CAD build for the part. Positions are in the model's coordinates, mm. Face numbers are marked on the shaded views. A direction names the side the tool comes from. Coordinates: 2 decimals unless noted, no trailing zeros. Loops run counter-clockwise (first coordinate to the right, second up) from the corner with the lowest first, then second, coordinate; pieces in that order, holes last. Notation, with made-up numbers: (54, 41.5) -> (76, 41.5) arc R23 cw to (76, 54.5) -> close; hole circle Ø10 at (64.5, 50.5). An arc over 180 degrees is marked (long way). Write each question's results on one line, items separated by ' | '.
from build123d import *

# Parameters (mm, degrees)
SKETCH_1_W          = 60
SKETCH_1_H          = 44
EXTRUDE_1_DEPTH     = 10
SKETCH_2_W          = 30
SKETCH_2_H          = 36
EXTRUDE_2_DEPTH     = 18
SKETCH_3_R          = 10
CUT_EXTRUDE_1_DEPTH = 47.561786907
RIB_1_REACH         = 48.562
SKETCH_5_WALL_W     = 123.548914622
SKETCH_5_WALL_H     = 6


with BuildPart() as part:
    # 草图1 → 凸台-拉伸1 (new body)
    with BuildSketch(Plane(origin=(0, 0, 0), x_dir=(1, 0, 0), z_dir=(0, 1, 0))):
        Rectangle(SKETCH_1_W, SKETCH_1_H)
    extrude(amount=EXTRUDE_1_DEPTH)

    # 草图2 → 凸台-拉伸2 (add)
    with BuildSketch(Plane(origin=(0, 10, 0), x_dir=(1, 0, 0), z_dir=(0, 1, 0))):
        with Locations((-7, 0)):
            Rectangle(SKETCH_2_W, SKETCH_2_H)
    extrude(amount=EXTRUDE_2_DEPTH)

    # 草图3 → 切除-拉伸1 (cut, through all)
    with BuildSketch(Plane(origin=(0, 28, 0), x_dir=(1, 0, 0), z_dir=(0, 1, 0))):
        with Locations(Location((-7, 0, 0), (0, 0, 270))):
            Circle(SKETCH_3_R)
    extrude(amount=-CUT_EXTRUDE_1_DEPTH, mode=Mode.SUBTRACT)

    # 草图5 wall → 筋1 (add, up to next)
    with BuildSketch(Plane(origin=(19, 19, 0), x_dir=(0.773957299203, -0.633237790257, 0), z_dir=(0.633237790257, 0.773957299203, 0)), mode=Mode.PRIVATE) as rib_1_sk1:
        Rectangle(SKETCH_5_WALL_W, SKETCH_5_WALL_H)
    rib_1_tool1 = extrude(rib_1_sk1.sketch, amount=-RIB_1_REACH, mode=Mode.PRIVATE) - part.part
    add(rib_1_tool1.solids().sort_by_distance((19, 19, 0))[0])


solid = part.part
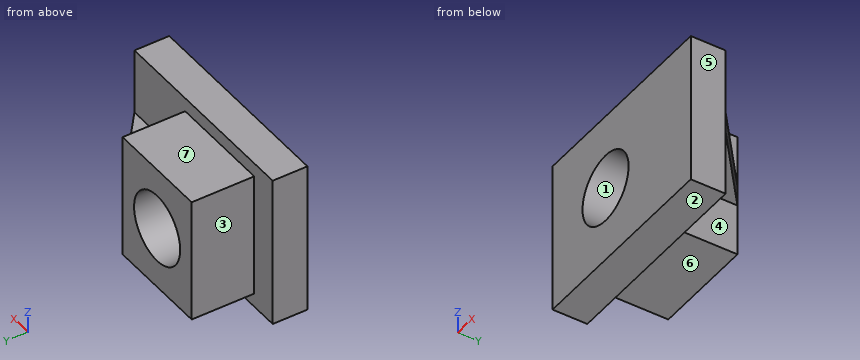
1) Two-plate mould, pull along X, no slides. Class the marked faces 1, 2 and 3: pulls with the +X half, pulls with the -X half, needs draft (parallel to the pull), parting line crosses it, or undercut.
Outcome:
face 1: undercut | face 2: needs draft | face 3: pulls with the -X half
2) Slice it at D-D (z = -11). Write the cut outline in (x, y).
Outcome:
outline: (-30, 0) -> (30, 0) -> (30, 10) -> (8, 10) -> (8, 28) -> (-22, 28) -> (-22, 10) -> (-30, 10) -> close
3) Drill centre lines: L1, parallel to Y at x = 9, z = 6.5; L2, parallel to Z at x = -21, y = 21; L3, parallel to X at y = 18.25, z = 7.5. Where is each one in solid material? Low to high. Write a range as from..to.
Outcome:
L1: y = 0..10 | L2: z = -18..18 | L3: x = -22..-13.61, -0.39..8
4) Slice it at A-A (z = 0). Write the cut outline in (x, y), then the cut area to 3 significant figures.
Outcome:
outline: (-30, 0) -> (-17, 0) -> (-17, 28) -> (-22, 28) -> (-22, 10) -> (-30, 10) -> close; (3, 0) -> (30, 0) -> (30, 10) -> (8, 28) -> (3, 28) -> close | area: 778 mm^2
5) Pin check, flat tips, straight feed: pin 1 (14.5 mm diameter, centred on x = 22.5, y = 22, fed in from -Z); pin 2 (5.5 mm diameter, centred on x = -13.5, y = 16.5, fed in from -Z); pin 3 (7.5 mm diameter, centred on y = 19.5, z = 11, fed in from +X); pin 4 (16 mm diameter, centred on x = -7, z = 0, fed in from +Y). Stop position of each tip, or through.
Outcome:
pin 1: stops at z = -3 | pin 2: stops at z = -18 | pin 3: stops at x = 8 | pin 4: passes through
6) Which spindle directions (+Z, -Z, +X, -X, +Y, -Y) get a long thin tool onto all of the face, cutting with end or side? Do the marked faces 4, 5, 6 and 7. Say none if no direction does.
Outcome:
face 4: -Z, +X, +Y | face 5: +Z, -Z, +X, +Y, -Y | face 6: -Z, +X, -X, +Y | face 7: +Z, +X, -X, +Y
7) Slice it at B-B (x = -7). Write the cut outline in (y, z), then the cut area to 3 significant figures.
Outcome:
outline: (0, -22) -> (10, -22) -> (10, -18) -> (28, -18) -> (28, -10) -> (0, -10) -> close; (0, 10) -> (28, 10) -> (28, 18) -> (10, 18) -> (10, 22) -> (0, 22) -> close | area: 528 mm^2
8) Slice it at C-C (y = 2.75). Write the cut outline in (x, z), then the cut area to 3 significant figures.
Outcome:
outline: (-30, -22) -> (30, -22) -> (30, 22) -> (-30, 22) -> close; hole circle Ø20 at (-7, 0) | area: 2,330 mm^2
